Read the model definition and answer for the solid it produces. Units are mm, in the model's axes. A direction names the side the tool comes from. Give positions to 0.01 mm unless a question says otherwise; leave off trailing zeros. Order: outer loops, then holes, each group sorted by start corner. A loop starts at its lowest first (then second) coordinate and runs counter-clockwise, first axis right, second up.
Item 1: A cutting plane is placed at A-A (x = 21.6). Write down the section's boundary in (y, z).
Item 2: Find the intervals of material crossed by line 1 along Y through (x, z) = (10, 31.5); line 2 along X through (y, z) = (2, 40), in increasing order.
Item 3: A cutting plane is placed at D-D (z = 22.5). Write down the section's boundary in (x, y), plus the area to 3 significant figures.
Item 4: Given pin 1 Ø0.8 at (y, z) = (2, 39.5) entering from +X; pin 2 Ø0.6 at (x, y) = (2.5, 2.5) entering from +Z; pin 3 Ø0.5 at (x, z) = (2, 38.5) entering from +Y, each flat-ended and moving along its own axis, determine where each tip first touches the part or whether it passes through.
Item 5: A cutting plane is placed at B-B (z = 39). Write down the section's boundary in (x, y), plus the area to 3 significant figures.
Item 6: Which of the six approach directions +Z, -Z, +X, -X, +Y, -Y give full straight-line access (tool end or side, diameter ignored) to faces 5 (the face through (39.39, 40.52, 33.83)), 6 (the face through (42.436, 42.476, 21.091)), 7 (the face through (4.316, 4.356, 38.029))?
Item 7: The mould has two halves that part along Z. Classify faces 1 (the face through (3.81, 40.52, 33.83)), 2 (the face through (16, 41, 0)), 3 (the face through (21, 43.2, 21)), 4 (the face through (3, 3, 36.6)): +Z half, -Z half, draft (parallel to the pull), parting line (faces both ways), or undercut.
Item 8: A cutting plane is placed at C-C (y = 34). Write down the section's boundary in (x, z), plus the area to 3 significant figures.
from build123d import *

# Parameters (mm, degrees)
CYLINDER001_R     = 2.4
CYLINDER001_DEPTH = 10
CYLINDER004_R     = 1
CYLINDER004_DEPTH = 5
CYLINDER005_R     = 1
CYLINDER005_DEPTH = 5
CYLINDER003_R     = 1
CYLINDER003_DEPTH = 5
CYLINDER002_R     = 1
CYLINDER002_DEPTH = 5
CYLINDER_R        = 19.4
CYLINDER_DEPTH    = 1.6
BOX004_W          = 5.08
BOX004_H          = 5.08
BOX004_DEPTH      = 10
CHAMFER_SIZE      = 3.5
FILLET002_R       = 2.54
BOX005_W          = 5.08
BOX005_H          = 5.08
BOX005_DEPTH      = 10
CHAMFER001_SIZE   = 3.5
FILLET003_R       = 2.54
BOX003_W          = 5.08
BOX003_H          = 5.08
BOX003_DEPTH      = 10
CHAMFER002_SIZE   = 3.5
FILLET004_R       = 2.54
BOX002_W          = 5.08
BOX002_H          = 5.08
BOX002_DEPTH      = 10
CHAMFER003_SIZE   = 3.5
FILLET001_R       = 2.54
BOX001_W          = 40
BOX001_H          = 40
BOX001_DEPTH      = 41.6
BOX_W             = 43.2
BOX_H             = 43.2
BOX_DEPTH         = 41.6
FILLET_R          = 0.94
FILLET005_R       = 2.54


with BuildPart() as ir:
    # Cylinder001 → Cylinder001 (new body)
    with BuildSketch(Plane(origin=(5.6, 5.6, 0), x_dir=(1, 0, 0), z_dir=(0, 0, 1))):
        Circle(CYLINDER001_R)
    extrude(amount=CYLINDER001_DEPTH)


with BuildPart() as zylinder002:
    # Cylinder004 → Cylinder004 (new body)
    with BuildSketch(Plane(origin=(2.54, 40.66, 36.6), x_dir=(1, 0, 0), z_dir=(0, 0, 1))):
        Circle(CYLINDER004_R)
    extrude(amount=CYLINDER004_DEPTH)


with BuildPart() as zylinder003:
    # Cylinder005 → Cylinder005 (new body)
    with BuildSketch(Plane(origin=(40.66, 40.66, 36.6), x_dir=(1, 0, 0), z_dir=(0, 0, 1))):
        Circle(CYLINDER005_R)
    extrude(amount=CYLINDER005_DEPTH)


with BuildPart() as zylinder001:
    # Cylinder003 → Cylinder003 (new body)
    with BuildSketch(Plane(origin=(40.66, 2.54, 36.6), x_dir=(1, 0, 0), z_dir=(0, 0, 1))):
        Circle(CYLINDER003_R)
    extrude(amount=CYLINDER003_DEPTH)


with BuildPart() as screws:
    # Cylinder002 → Cylinder002 (new body)
    with BuildSketch(Plane(origin=(2.54, 2.54, 36.6), x_dir=(1, 0, 0), z_dir=(0, 0, 1))):
        Circle(CYLINDER002_R)
    extrude(amount=CYLINDER002_DEPTH)

    # Fusion002: union Zylinder002, Zylinder003, Zylinder001
    add(zylinder002.part)
    add(zylinder003.part)
    add(zylinder001.part)


with BuildPart() as speaker:
    # Cylinder → Cylinder (new body)
    with BuildSketch(Plane(origin=(21.6, 21.6, 0), x_dir=(1, 0, 0), z_dir=(0, 0, 1))):
        Circle(CYLINDER_R)
    extrude(amount=CYLINDER_DEPTH)


with BuildPart() as fillet002:
    # Box004 → Box004 (new body)
    with BuildSketch(Plane(origin=(0, 38.12, 31.6), x_dir=(1, 0, 0), z_dir=(0, 0, 1))):
        with Locations((2.54, 2.54)):
            Rectangle(BOX004_W, BOX004_H)
    extrude(amount=BOX004_DEPTH)

    # Chamfer
    chamfer_edges = [fillet002.edges().sort_by_distance(p)[0] for p in [
        (5.08, 40.66, 31.6),
        (2.54, 38.12, 31.6),
    ]]
    chamfer(chamfer_edges, length=CHAMFER_SIZE)

    # Fillet002
    fillet002_edges = [fillet002.edges().sort_by_distance(p)[0] for p in [
        (5.08, 38.12, 38.35),
    ]]
    fillet(fillet002_edges, radius=FILLET002_R)


with BuildPart() as fillet003:
    # Box005 → Box005 (new body)
    with BuildSketch(Plane(origin=(38.12, 38.12, 31.6), x_dir=(1, 0, 0), z_dir=(0, 0, 1))):
        with Locations((2.54, 2.54)):
            Rectangle(BOX005_W, BOX005_H)
    extrude(amount=BOX005_DEPTH)

    # Chamfer001
    chamfer001_edges = [fillet003.edges().sort_by_distance(p)[0] for p in [
        (38.12, 40.66, 31.6),
        (40.66, 38.12, 31.6),
    ]]
    chamfer(chamfer001_edges, length=CHAMFER001_SIZE)

    # Fillet003
    fillet003_edges = [fillet003.edges().sort_by_distance(p)[0] for p in [
        (38.12, 38.12, 38.35),
    ]]
    fillet(fillet003_edges, radius=FILLET003_R)


with BuildPart() as fillet004:
    # Box003 → Box003 (new body)
    with BuildSketch(Plane(origin=(38.12, 0, 31.6), x_dir=(1, 0, 0), z_dir=(0, 0, 1))):
        with Locations((2.54, 2.54)):
            Rectangle(BOX003_W, BOX003_H)
    extrude(amount=BOX003_DEPTH)

    # Chamfer002
    chamfer002_edges = [fillet004.edges().sort_by_distance(p)[0] for p in [
        (38.12, 2.54, 31.6),
        (40.66, 5.08, 31.6),
    ]]
    chamfer(chamfer002_edges, length=CHAMFER002_SIZE)

    # Fillet004
    fillet004_edges = [fillet004.edges().sort_by_distance(p)[0] for p in [
        (38.12, 5.08, 38.35),
    ]]
    fillet(fillet004_edges, radius=FILLET004_R)


with BuildPart() as holder:
    # Box002 → Box002 (new body)
    with BuildSketch(Plane.XY.offset(31.6)):
        with Locations((2.54, 2.54)):
            Rectangle(BOX002_W, BOX002_H)
    extrude(amount=BOX002_DEPTH)

    # Chamfer003
    chamfer003_edges = [holder.edges().sort_by_distance(p)[0] for p in [
        (5.08, 2.54, 31.6),
        (2.54, 5.08, 31.6),
    ]]
    chamfer(chamfer003_edges, length=CHAMFER003_SIZE)

    # Fillet001
    fillet001_edges = [holder.edges().sort_by_distance(p)[0] for p in [
        (5.08, 5.08, 38.35),
    ]]
    fillet(fillet001_edges, radius=FILLET001_R)

    # Fusion: union Fillet002, Fillet003, Fillet004
    add(fillet002.part)
    add(fillet003.part)
    add(fillet004.part)


with BuildPart() as obj1:
    # Box001 → Box001 (new body)
    with BuildSketch(Plane(origin=(1.6, 1.6, 1.6), x_dir=(1, 0, 0), z_dir=(0, 0, 1))):
        with Locations((20, 20)):
            Rectangle(BOX001_W, BOX001_H)
    extrude(amount=BOX001_DEPTH)


with BuildPart() as cut003:
    # Box → Box (new body)
    with BuildSketch(Plane.XY):
        with Locations((21.6, 21.6)):
            Rectangle(BOX_W, BOX_H)
    extrude(amount=BOX_DEPTH)

    # Cut: cut obj1
    add(obj1.part, mode=Mode.SUBTRACT)

    # Fillet
    fillet_edges = [cut003.edges().sort_by_distance(p)[0] for p in [
        (41.6, 1.6, 21.6),
        (41.6, 41.6, 21.6),
        (1.6, 41.6, 21.6),
        (1.6, 1.6, 21.6),
    ]]
    fillet(fillet_edges, radius=FILLET_R)

    # Fusion001: union Holder
    add(holder.part)

    # Fillet005
    fillet005_edges = [cut003.edges().sort_by_distance(p)[0] for p in [
        (0, 0, 15.8),
        (0, 43.2, 15.8),
        (43.2, 43.2, 15.8),
        (43.2, 0, 15.8),
        (0, 0, 36.6),
        (0, 43.2, 36.6),
        (43.2, 43.2, 36.6),
        (43.2, 0, 36.6),
    ]]
    fillet(fillet005_edges, radius=FILLET005_R)

    # Cut001: cut Speaker
    add(speaker.part, mode=Mode.SUBTRACT)

    # Cut002: cut Screws
    add(screws.part, mode=Mode.SUBTRACT)

    # Cut003: cut IR
    add(ir.part, mode=Mode.SUBTRACT)


solid = cut003.part
Response values:
1. outline: (0, 0) - (2.2, 0) - (2.2, 1.6) - (1.6, 1.6) - (1.6, 41.6) - (0, 41.6) - close; (41, 0) - (43.2, 0) - (43.2, 41.6) - (41.6, 41.6) - (41.6, 1.6) - (41, 1.6) - close
2. line 1: y = 0 to 1.6, 41.6 to 43.2
2. line 2: x = 0.06 to 1.7, 3.38 to 5.08, 38.12 to 39.82, 41.5 to 43.14
3. outline: (0, 2.54) arc R2.54 ccw to (2.54, 0) - (40.66, 0) arc R2.54 ccw to (43.2, 2.54) - (43.2, 40.66) arc R2.54 ccw to (40.66, 43.2) - (2.54, 43.2) arc R2.54 ccw to (0, 40.66) - close; hole (1.6, 2.54) arc R0.94 ccw to (2.54, 1.6) - (40.66, 1.6) arc R0.94 ccw to (41.6, 2.54) - (41.6, 40.66) arc R0.94 ccw to (40.66, 41.6) - (2.54, 41.6) arc R0.94 ccw to (1.6, 40.66) - close
3. area: 261 mm2
4. pin 1: stops at x = 43.2
4. pin 2: stops at z = 36.6
4. pin 3: stops at y = 43.18
5. outline: (0, 2.54) arc R2.54 ccw to (2.54, 0) - (40.66, 0) arc R2.54 ccw to (43.2, 2.54) - (43.2, 40.66) arc R2.54 ccw to (40.66, 43.2) - (2.54, 43.2) arc R2.54 ccw to (0, 40.66) - close; hole circle Ø2 at (2.54, 2.54); hole circle Ø2 at (2.54, 40.66); hole (1.6, 5.08) - (2.54, 5.08) arc R2.54 cw to (5.08, 2.54) - (5.08, 1.6) - (38.12, 1.6) - (38.12, 2.54) arc R2.54 cw to (40.66, 5.08) - (41.6, 5.08) - (41.6, 38.12) - (40.66, 38.12) arc R2.54 cw to (38.12, 40.66) - (38.12, 41.6) - (5.08, 41.6) - (5.08, 40.66) arc R2.54 cw to (2.54, 38.12) - (1.6, 38.12) - close; hole circle Ø2 at (40.66, 2.54); hole circle Ø2 at (40.66, 40.66)
5. area: 291 mm2
6. face 5: none
6. face 6: +Z, -Z, +X, +Y
6. face 7: +Z
7. face 1: undercut
7. face 2: -Z half
7. face 3: draft
7. face 4: +Z half
8. outline: (0, 0) - (6.68, 0) - (6.68, 1.6) - (1.6, 1.6) - (1.6, 41.6) - (0, 41.6) - close; (36.52, 0) - (43.2, 0) - (43.2, 41.6) - (41.6, 41.6) - (41.6, 1.6) - (36.52, 1.6) - close
8. area: 149 mm2
